Build history of the part. All positions in model axes, mm. Face numbers are marked on the shaded views. A direction names the side the tool comes from. Coordinates: 2 decimals unless noted, no trailing zeros. Write each loop counter-clockwise with the first axis right and the second up, starting at its lowest first coordinate (ties: lowest second). Pieces come first, ordered by that corner, then holes.
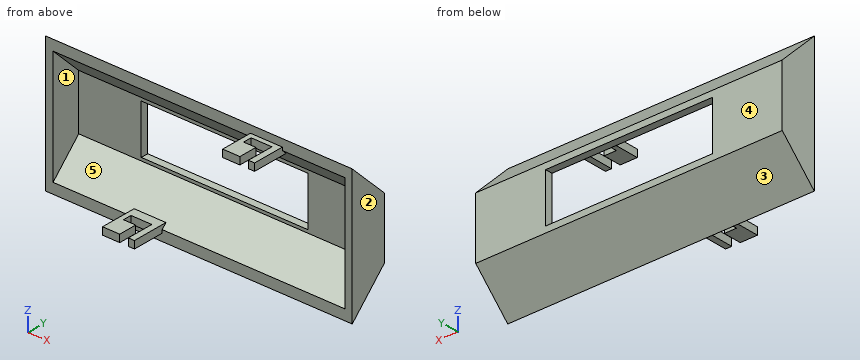
from build123d import *

# Parameters (mm, degrees)
SKETCH1_W           = 125
SKETCH1_H           = 55
BOSS_EXTRUDE1_DEPTH = 15
CHAMFER1_SIZE       = 15
SHELL1_START        = 3
SHELL1_DEPTH        = 119
SKETCH2_W           = 13
SKETCH2_H           = 3
BOSS_EXTRUDE3_DEPTH = 13
SKETCH3_W           = 3.5
SKETCH3_H           = 7.5
SKETCH3_W_2         = 8.5
SKETCH3_H_2         = 3.5
CUT_EXTRUDE1_DEPTH  = 13
SKETCH5_W           = 3.5
SKETCH5_H           = 7.5
SKETCH5_W_2         = 8.5
SKETCH5_H_2         = 3.5
CUT_EXTRUDE2_DEPTH  = 13
SKETCH6_W           = 68
SKETCH6_H           = 20
CUT_EXTRUDE3_DEPTH  = 3
SKETCH7_W           = 13
SKETCH7_H           = 1.757359313
BOSS_EXTRUDE4_DEPTH = 4
SKETCH8_W           = 13
SKETCH8_H           = 1.757359313
BOSS_EXTRUDE5_DEPTH = 4


# Read off the part's stored shape, not the designer's step: Shell1
with BuildPart() as part:
    # Sketch1 → Boss-Extrude1 (new body)
    with BuildSketch(Plane(origin=(0, 0, 0), x_dir=(1, 0, 0), z_dir=(0, 1, 0))):
        with Locations((62.5, -27.5)):
            Rectangle(SKETCH1_W, SKETCH1_H)
    extrude(amount=BOSS_EXTRUDE1_DEPTH)

    # Chamfer1
    chamfer1_edges = [part.edges().sort_by_distance(p)[0] for p in [
        (62.5, 15, 55),
        (62.5, 15, 0),
    ]]
    chamfer(chamfer1_edges, length=CHAMFER1_SIZE - 0.0001)  # a hair under: the kernel refuses the full size

    # Shell1 outline → Shell1 (cut)
    with BuildSketch(Plane.YZ.offset(SHELL1_START)):
        Polygon((0, 4.242640687), (12, 16.242640687), (12, 38.757359313), (0, 50.757359313), align=None)
    extrude(amount=SHELL1_DEPTH, mode=Mode.SUBTRACT)

    # Sketch2 → Boss-Extrude3 (add)
    with BuildSketch(Plane(origin=(0, 0, 0), x_dir=(-1, 0, 0), z_dir=(0, -1, 0))):
        with Locations((-41, -4.5)):
            Rectangle(SKETCH2_W, SKETCH2_H)
        with Locations((-90, -50.5)):
            Rectangle(SKETCH2_W, SKETCH2_H)
    extrude(amount=BOSS_EXTRUDE3_DEPTH)

    # Sketch3 → Cut-Extrude1 (cut)
    with BuildSketch(Plane.XY.offset(52)):
        with Locations((92.25, -9.25)):
            Rectangle(SKETCH3_W, SKETCH3_H)
        with Locations((89.75, -3.75)):
            Rectangle(SKETCH3_W_2, SKETCH3_H_2)
    extrude(amount=-CUT_EXTRUDE1_DEPTH, mode=Mode.SUBTRACT)

    # Sketch5 → Cut-Extrude2 (cut)
    with BuildSketch(Plane(origin=(0, 0, 3), x_dir=(-1, 0, 0), z_dir=(0, 0, -1))):
        with Locations((-43.25, -9.25)):
            Rectangle(SKETCH5_W, SKETCH5_H)
        with Locations((-40.75, -3.75)):
            Rectangle(SKETCH5_W_2, SKETCH5_H_2)
    extrude(amount=-CUT_EXTRUDE2_DEPTH, mode=Mode.SUBTRACT)

    # Sketch6 → Cut-Extrude3 (cut)
    with BuildSketch(Plane(origin=(0, 15, 0), x_dir=(1, 0, 0), z_dir=(0, 1, 0))):
        with Locations((62.5, -27.5)):
            Rectangle(SKETCH6_W, SKETCH6_H)
    extrude(amount=-CUT_EXTRUDE3_DEPTH, mode=Mode.SUBTRACT)

    # Sketch7 → Boss-Extrude4 (add)
    with BuildSketch(Plane(origin=(0, 0, 0), x_dir=(1, 0, 0), z_dir=(0, 1, 0))):
        with Locations((41, -5.121320344)):
            Rectangle(SKETCH7_W, SKETCH7_H)
    extrude(amount=BOSS_EXTRUDE4_DEPTH)

    # Sketch8 → Boss-Extrude5 (add)
    with BuildSketch(Plane(origin=(0, 0, 0), x_dir=(1, 0, 0), z_dir=(0, 1, 0))):
        with Locations((90, -49.878679656)):
            Rectangle(SKETCH8_W, SKETCH8_H)
    extrude(amount=BOSS_EXTRUDE5_DEPTH)


solid = part.part
(1) Slice it at C-C, the plane y = -4. List the corners of the cut face in (x, z), and give its area (3 significant figures).
(2) Slice it at D-D, the plane y = 8.25. List the corners of the cut face in (x, z).
(3) Slice it at A-A, the plane z = 34. List the corners of the cut face in (x, y).
(4) Probe L1, parallel to X at y = 7.75, z = 23.5; L2, parallel to Y at x = 5.5, z = 29; L3, parallel to Z at x = 97, y = 6. List the from-to ranges inside material, lowest first.
(5) Flat gauge pins, fed straight in: P1, Ø4, axis at x = 39, y = -3, coming from the +Z side; P2, Ø10.5, axis at x = 92, y = -7.5, coming from the -Z side; P3, Ø0.9, axis at x = 87, z = 51, coming from the +Y side. Where does each tip first touch, or does it go through?
(6) Two-plate mould, pull along X, no slides. Class the marked faces 1, 2 and 3: pulls with the +X half, pulls with the -X half, needs draft (parallel to the pull), parting line crosses it, or undercut.
(7) 3-axis set-ups, long thin cutter, end or side, ignore diameter. For the marked faces 4 and 5: which of +Z, -Z, +X, -X, +Y, -Y reach the whole face in a straight line?
Results:
1. outline: (34.5, 3) - (36.5, 3) - (36.5, 6) - (34.5, 6) - close; (45, 3) - (47.5, 3) - (47.5, 6) - (45, 6) - close; (83.5, 49) - (85.5, 49) - (85.5, 52) - (83.5, 52) - close; (94, 49) - (96.5, 49) - (96.5, 52) - (94, 52) - close
1. area: 27.0 mm2
2. outline: (0, 8.25) - (125, 8.25) - (125, 46.75) - (0, 46.75) - close; hole (3, 12.49) - (122, 12.49) - (122, 42.51) - (3, 42.51) - close
3. outline: (0, 0) - (3, 0) - (3, 12) - (28.5, 12) - (28.5, 15) - (0, 15) - close; (96.5, 12) - (122, 12) - (122, 0) - (125, 0) - (125, 15) - (96.5, 15) - close
4. L1: x = 0 to 3, 122 to 125
4. L2: y = 12 to 15
4. L3: z = 6 to 10.24, 44.76 to 49
5. P1: stops at z = 6
5. P2: stops at z = 49
5. P3: stops at y = 4.45
6. face 1: undercut
6. face 2: pulls with the +X half
6. face 3: needs draft
7. face 4: +Z, -Z, +X, -X, +Y
7. face 5: -Y
